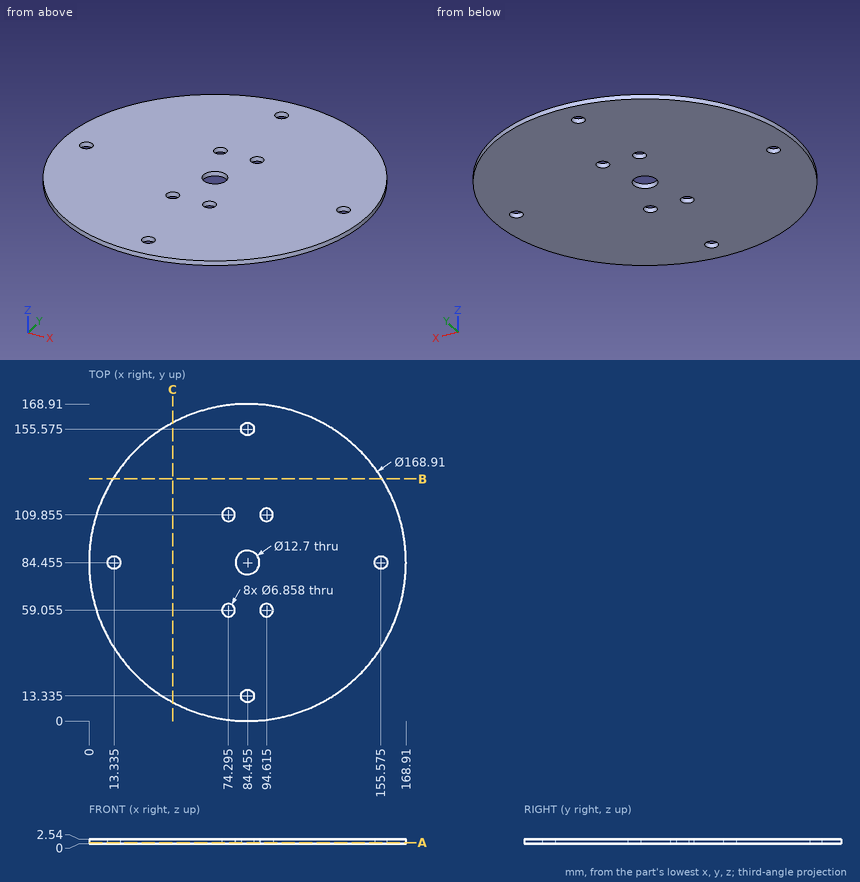
The drawing under review shows one solid part. Ordinate dimensions are in mm from its lowest x, y, z. Give positions to 0.01 mm unless a question says otherwise; leave off trailing zeros. Write each loop counter-clockwise with the first axis right and the second up, starting at its lowest first coordinate (ties: lowest second). Pieces come first, ordered by that corner, then holes. Notation, with made-up numbers: (-17.75, -12) -> (11.25, -12) arc R18 cw to (11.25, 12) -> close; hole circle Ø3 at (-31.75, -2.5). An arc over 180 degrees is marked (long way). Put each result on its own line as item: value.
(1) To check wall thickness, follow probe 1 along X at (y, z) = (83, 1.2); probe 2 along X at (y, z) = (57.5, 2.2); probe 3 along Y at (x, z) = (87.5, 1.25). State the ranges of each line that lie inside material, in increasing order. Write a range as from..to.
Results are:
probe 1: 0.01..10.23, 16.44..78.27, 90.64..152.47, 158.68..168.9
probe 2: 4.42..71.24, 77.35..91.56, 97.67..164.49
probe 3: 0.05..11.76, 14.91..78.88, 90.03..154, 157.15..168.86
(2) We need section B-B, the plane y = 129. Give the boundary of the cut face in (x, z), and give its area (3 significant figures).
Results are:
outline: (12.7, 0) -> (156.21, 0) -> (156.21, 2.54) -> (12.7, 2.54) -> close
area: 365 mm²
(3) We need section A-A, the plane z = 0.55. State how many separate pieces and enclosed holes the cut face has, and give its area (3 significant figures).
Results are:
separate pieces: 1
enclosed holes: 9
area: 22,000 mm²
(4) For pin 1 Ø5.5 at (x, y) = (84.455, 13.335) entering from -Z, flat-tipped, find the tip position at first contact; note if it passes through.
Results are:
pin 1: through
(5) We need section C-C, the plane x = 44.5. Give the boundary of the cut face in (y, z), and give its area (3 significant figures).
Results are:
outline: (10.05, 0) -> (158.86, 0) -> (158.86, 2.54) -> (10.05, 2.54) -> close
area: 378 mm²
